Work out the finished part from the listing and answer in its coordinate system (mm). Round coordinates to 2 decimals unless told otherwise and drop trailing zeros. Order: outer loops, then holes, each group sorted by start corner. A loop starts at its lowest first (then second) coordinate and runs counter-clockwise, first axis right, second up. Notation, with made-up numbers: M 85,76 L 100,76 A31 cw 100,105 Z; hole C 56,1.5 d3. An arc over 180 degrees is marked long. Answer as a JSON object with one key per item and string values. Group by question number.
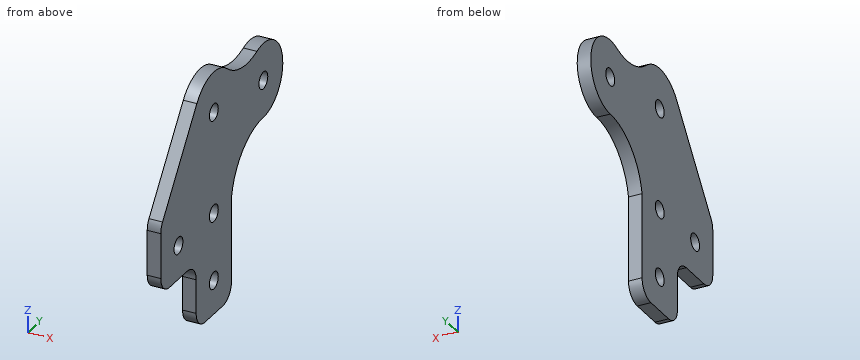
Autodesk Inventor part; units mm, degrees
ref_plane "YZ Plane" through (0, 0, 0) normal (1, 0, 0) x (0, 1, 0)
ref_plane "XZ Plane" through (0, 0, 0) normal (0, 1, 0) x (-1, 0, 0)
ref_plane "XY Plane" through (0, 0, 0) normal (0, 0, 1) x (1, 0, 0)
sketch "Skizze1" plane through (0, 0, 0) normal (1, 0, 0) x (0, 1, 0)
  line L0 (-30, 10) -> (-30, -10)
  arc A0 (28, 15) -> (24.3693, 36.3836) centre (28, 26) ccw
  line L1 (-9.6, 37.2) -> (-30, 10)
  line L2 (10, -3) -> (10, 0)
  arc A1 (28, 15) -> (10, 0) centre (28, -3.3) ccw
  line L3 (-10, -30) -> (10, -30)
  line L4 (10, -30) -> (10, 0)
  line L5 (-10, -10) -> (-30, -10)
  line L6 (-10, -10) -> (-10, -30)
  arc A2 (7.5634, 39.3164) -> (24.3693, 36.3836) centre (18.5933, 52.9028) ccw
  arc A3 (7.5634, 39.3164) -> (-9.6, 37.2) centre (0, 30) ccw
  point P0 (0, 0)
  point P1 (-30, 0)
  dimension "d16" = 22
  dimension "d22" = 10
  dimension "d23" = 18
  dimension "d26" = 30
  dimension "d31" = 20
  dimension "d34" = 26
  dimension "d35" = 10
  dimension "d36" = 20
  dimension "d37" = 18
  dimension "d38" = 18
  dimension "d39" = 0
  dimension "d40" = 30
  dimension "d43" = 35
  dimension "d44" = 12
  dimension "d46" = 0
extrude "Extrusion1" add sketch "Skizze1" along normal mid plane 4
sketch "Skizze2" plane through (2, 0, 0) normal (1, 0, 0) x (0, 0, -1)
  circle A0 centre (-26, 28) radius 2.5
  circle A1 centre (0, 0) radius 2.5
  circle A2 centre (20, 0) radius 2.5
  circle A3 centre (0, -20) radius 2.5
  line L0 (-10, -30) -> (10, -30)
  line L1 (30, -10) -> (30, 10)
  arc A4 (-15, 28) -> (-36.3836, 24.3693) centre (-26, 28) ccw
  circle A5 centre (-30, 0) radius 2.5
  arc A6 (-39.3164, 7.5634) -> (-37.2, -9.6) centre (-30, 0) ccw
  point P0 (10, -27)
  point P1 (-36.9988, 28.1611)
  point P2 (-44.9983, -10.001)
  dimension "d8" = 5
  dimension "d9" = 5
  dimension "d10" = 5
  dimension "d11" = 10
  dimension "d32" = 10
  dimension "d45" = 5
extrude "Extrusion2" cut sketch "Skizze2" along normal through all both and the other way through all
fillet "Fillet1" radius 5 5 edges at (0, -30, -10) (0, -10, -10) (0, -10, -30) (0, 10, -30) (0, -30, 10)
properties part number "KettenBlech_Oben"
Item 1: Find section A-A (y = 0). Give the vertices of the cut face in (x, z).
Item 2: Each of these flat-tipped pins is pushed along its axis until it touches: pin 1 (1 mm diameter, centred on x = 0.5, z = -13, fed in from -Y); pin 2 (1.5 mm diameter, centred on x = 1.5, z = -22, fed in from +Y); pin 3 (2 mm diameter, centred on x = 1, z = -22, fed in from -Y). Where does it stop, or does it pass through?
Item 3: Find section B-B (z = 26). Give the vertices of the cut face in (x, y).
Item 4: Find section C-C (x = 0.2). Give the vertices of the cut face in (y, z), and give its area (3 significant figures).
Item 5: Consider L1, parallel to Y at x = -0.5, z = -15.5; L2, parallel to Z at x = 1, y = 29; L3, parallel to Y at x = -0.45, z = 30. Determine where each line is inside the solid, lowest interval first.
Item 6: Find section D-D (z = -20). Give the vertices of the cut face in (x, y).
Responses:
{
 "1": {"outline": "M -2,-30 L 2,-30 L 2,-22.5 L -2,-22.5 Z; M -2,-17.5 L 2,-17.5 L 2,-2.5 L -2,-2.5 Z; M -2,2.5 L 2,2.5 L 2,27.5 L -2,27.5 Z; M -2,32.5 L 2,32.5 L 2,42 L -2,42 Z"},
 "2": {"pin 1": "stops at y = -10.67", "pin 2": "stops at y = 10", "pin 3": "stops at y = -10"},
 "3": {"outline": "M -2,-18 L 2,-18 L 2,25.5 L -2,25.5 Z; M -2,30.5 L 2,30.5 L 2,39 L -2,39 Z"},
 "4": {"outline": "M -30,-5 A5 ccw -25,-10 L -15,-10 A5 cw -10,-15 L -10,-25 A5 ccw -5,-30 L 5,-30 A5 ccw 10,-25 L 10,0 A18.3 cw 28,15 A11 ccw long 24.37,36.38 A17.5 cw 7.56,39.32 A12 ccw -9.6,37.2 L -29,11.33 A5 ccw -30,8.33 Z; hole C -20,0 d5; hole C 0,-20 d5; hole C 0,0 d5; hole C 0,30 d5; hole C 28,26 d5", "area": "2,600 mm^2"},
 "5": {"L1": "y = -10 to 10", "L2": "z = 15.05 to 23.71, 28.29 to 36.95", "L3": "y = -15 to -2.5, 2.5 to 38.25"},
 "6": {"outline": "M -2,-10 L 2,-10 L 2,-2.5 L -2,-2.5 Z; M -2,2.5 L 2,2.5 L 2,10 L -2,10 Z"}
}
